Geometry: final body of the model. Coordinates: model frame, mm. Give positions to 0.01 mm unless a question says otherwise; leave off trailing zeros. Write each loop counter-clockwise with the first axis right and the second up, starting at its lowest first coordinate (ties: lowest second). Pieces come first, ordered by that corner, then holes. Notation, with made-up numbers: M 74.25,49.5 L 85.25,49.5 A20 ccw 85.25,65.5 Z; hole C 32.25,-39.75 d2. An arc over 180 degrees is marked long. Answer as a JSON object with one key per item and string values.
from build123d import *

# Parameters (mm, degrees)
F3_DEPTH = 50.8
F4_DEPTH = 25.4
F5_R     = 11.945502
F6_DEPTH = 25.401
F7_R     = 13.410592
F8_DEPTH = 50.801


with BuildPart() as f3:
    # F2 (on face) → F3 (new body)
    with BuildSketch(Plane.XZ):
        with BuildLine():
            Line((42.025454, -24.601573), (42.025454, 24.601573))
            ThreePointArc((42.025454, 24.601573), (17.423881, 0), (42.025454, -24.601573))
        make_face()
        with BuildLine():
            ThreePointArc((42.025454, -24.601573), (59.421394, -17.395939), (66.627028, 0))
            ThreePointArc((66.627028, 0), (59.421394, 17.395939), (42.025454, 24.601573))
            Line((42.025454, 24.601573), (42.025454, -24.601573))
        make_face()
    extrude(amount=F3_DEPTH)

    # F1 (on face) → F4 (join)
    with BuildSketch(Plane.XZ):
        with BuildLine():
            ThreePointArc((-42.025454, 24.720491), (-24.545428, 17.480027), (-17.304963, 0))
            ThreePointArc((-17.304963, 0), (-24.545428, -17.480027), (-42.025454, -24.720491))
            Line((-42.025454, -24.720491), (-42.025454, -24.822727))
            Line((-42.025454, -24.822727), (42.025454, -24.822727))
            Line((42.025454, -24.822727), (42.025454, 24.822727))
            Line((42.025454, 24.822727), (-42.025454, 24.822727))
            Line((-42.025454, 24.822727), (-42.025454, 24.720491))
        make_face()
        with BuildLine():
            Line((-42.025454, -24.720491), (-42.025454, 24.720491))
            ThreePointArc((-42.025454, 24.720491), (-66.745945, 0), (-42.025454, -24.720491))
        make_face()
        with BuildLine():
            ThreePointArc((-42.025454, -24.720491), (-24.545428, -17.480027), (-17.304963, 0))
            ThreePointArc((-17.304963, 0), (-24.545428, 17.480027), (-42.025454, 24.720491))
            Line((-42.025454, 24.720491), (-42.025454, -24.720491))
        make_face()
    extrude(amount=F4_DEPTH)

    # F5 (on face) → F6 (cut, through all)
    with BuildSketch(Plane.XZ.offset(25.4)):
        with Locations((-42.025454, 0)):
            Circle(F5_R)
    extrude(amount=-F6_DEPTH, mode=Mode.SUBTRACT)

    # F7 (on face) → F8 (cut, through all)
    with BuildSketch(Plane.XZ.offset(50.8)):
        with Locations((42.025454, 0)):
            Circle(F7_R)
    extrude(amount=-F8_DEPTH, mode=Mode.SUBTRACT)


solid = f3.part
1) Cut plane A-A on z = 2. Return loops of the section in (x, y).
Geometry check:
{"outline": "M -66.66,-25.4 L -53.8,-25.4 L -53.8,0 L -66.66,0 Z; M -30.25,-25.4 L 17.51,-25.4 L 17.51,-50.8 L 28.76,-50.8 L 28.76,0 L -30.25,0 Z; M 55.29,-50.8 L 66.55,-50.8 L 66.55,0 L 55.29,0 Z"}
2) Cut plane B-B on y = -15. Return loops of the section in (x, z).
Geometry check:
{"outline": "M -42.03,-24.82 L 42.03,-24.82 L 42.03,-24.6 A24.6 ccw 42.03,24.6 L 42.03,24.82 L -42.03,24.82 L -42.03,24.72 A24.72 ccw -42.03,-24.72 Z; hole C -42.03,0 d23.89; hole C 42.03,0 d26.82"}
3) Cut plane D-D on z = 17.5. Return loops of the section in (x, y), and give its area (3 significant figures).
Geometry check:
{"outline": "M -59.49,-25.4 L 24.73,-25.4 L 24.73,-50.8 L 59.32,-50.8 L 59.32,0 L -59.49,0 Z", "area": "3,900 mm2"}
4) Line query: line 1 (X direction, y = -20.5, z = 0.5); line 2 (X direction, y = -16.5, z = 3); line 3 (Y direction, x = -43, z = 19.5). Output: solid intervals per line, ascending. Write a range as from..to.
Geometry check:
{"line 1": "x = -66.74..-53.96, -30.09..28.62, 55.43..66.62", "line 2": "x = -66.56..-53.59, -30.46..28.95, 55.1..66.44", "line 3": "y = -25.4..0"}
5) Contact query for flat-ended pins moving along their axis: P1, Ø19, axis at x = -42.03, z = 0, coming from the +Y side; P2, Ø2, axis at y = -30.5, z = 6.5, coming from the +X side; P3, Ø6, axis at x = 27, y = -37.5, coming from the +Z side; P4, Ø3, axis at y = -43.5, z = -7, coming from the -X side. Output: stop coordinate, or through.
Geometry check:
{"P1": "passes through", "P2": "stops at x = 66", "P3": "stops at z = 21.46", "P4": "stops at x = 18.05"}
6) Pull-direction query (X, two-part tool) for faces 1 (the cylindrical face through (28.628, -25.756, 0.59)), 2 (the cylindrical face through (-53.96, -12.88, 0.53)), 3 (the flat face through (-1, 0, 0)), 4 (the cylindrical face through (-66.74, -12.52, 0.54)); classes: pulls with the +X half, pulls with the -X half, needs draft (parallel to the pull), parting line crosses it, or undercut.
Geometry check:
{"face 1": "undercut", "face 2": "undercut", "face 3": "needs draft", "face 4": "pulls with the -X half"}
7) Cut plane C-C on x = -44. Return loops of the section in (y, z), and give its area (3 significant figures).
Geometry check:
{"outline": "M -25.4,-24.64 L 0,-24.64 L 0,-11.78 L -25.4,-11.78 Z; M -25.4,11.78 L 0,11.78 L 0,24.64 L -25.4,24.64 Z", "area": "653 mm2"}
